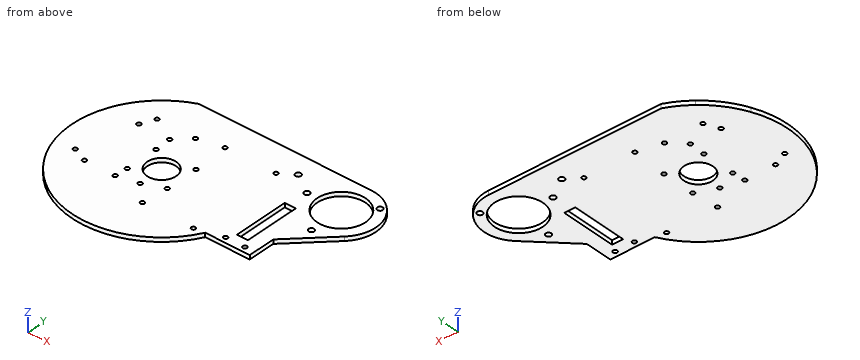
from build123d import *

# Parameters (mm, degrees)
SKETCH1_R           = 10.5
SKETCH1_R_2         = 1.5
SKETCH1_W           = 8
SKETCH1_H           = 40
SKETCH1_R_3         = 17.5
BOSS_EXTRUDE1_DEPTH = 3
CUT_EXTRUDE1_REACH  = 140.687
SKETCH2_R           = 2
CUT_EXTRUDE2_REACH  = 140.687
SKETCH3_R           = 2
BOSS_EXTRUDE2_START = -3
SKETCH4_R           = 65
SKETCH4_R_2         = 60
BOSS_EXTRUDE2_DEPTH = 3
CUT_EXTRUDE3_START  = -10
CUT_EXTRUDE3_DEPTH  = 10
CUT_EXTRUDE4_START  = -10
CUT_EXTRUDE4_DEPTH  = 10
CUT_EXTRUDE5_REACH  = 142.922
SKETCH7_R           = 1.5
CUT_EXTRUDE6_REACH  = 142.922
SKETCH8_R           = 1.5
CUT_EXTRUDE7_REACH  = 142.922
SKETCH9_R           = 1.5


with BuildPart() as part:
    # Sketch1 → Boss-Extrude1 (new body)
    # profile 1 of 2: a face of its own
    with BuildSketch(Plane.XY):
        with BuildLine():
            ThreePointArc((-60, 0), (-52.867640737, 28.372743309), (-33.166247904, 50))
            Line((-33.166247904, 50), (-60, 50))
            Line((-60, 50), (-60, 0))
        make_face()
    # profile 2 of 2: a face of its own
    with BuildSketch(Plane.XY):
        with BuildLine():
            ThreePointArc((0, 60), (-17.320508076, 57.445626465), (-33.166247904, 50))
            ThreePointArc((-33.166247904, 50), (-52.867640737, 28.372743309), (-60, 0))
            ThreePointArc((-60, 0), (-15.529142706, -57.955549577), (51.961524227, -30))
            Line((51.961524227, -30), (56.568542495, -30))
            Line((56.568542495, -30), (90, -30))
            Line((90, -30), (90, -10.355339059))
            Line((90, -10.355339059), (117.67766953, 17.32233047))
            ThreePointArc((117.67766953, 17.32233047), (123.096988313, 44.567085809), (100, 60))
            Line((100, 60), (0, 60))
        make_face()
        Circle(SKETCH1_R, mode=Mode.SUBTRACT)
        with Locations((69, -26)):
            Circle(SKETCH1_R_2, mode=Mode.SUBTRACT)
        with Locations((76, 0)):
            Rectangle(SKETCH1_W, SKETCH1_H, mode=Mode.SUBTRACT)
        with Locations((83, -26)):
            Circle(SKETCH1_R_2, mode=Mode.SUBTRACT)
        with Locations((100, 35)):
            Circle(SKETCH1_R_3, mode=Mode.SUBTRACT)
    extrude(amount=BOSS_EXTRUDE1_DEPTH)

    # Sketch2 → Cut-Extrude1 (cut, up to next)
    with BuildSketch(Plane.XY.offset(3), mode=Mode.PRIVATE) as cut_extrude1_sk1:
        with Locations((60, 45)):
            Circle(SKETCH2_R)
    cut_extrude1_tool1 = extrude(cut_extrude1_sk1.sketch, amount=-CUT_EXTRUDE1_REACH, mode=Mode.PRIVATE) & part.part
    add(cut_extrude1_tool1.solids().sort_by_distance((60, 45, 3))[0], mode=Mode.SUBTRACT)

    # Sketch3 → Cut-Extrude2 (cut, up to next)
    with BuildSketch(Plane.XY.offset(3), mode=Mode.PRIVATE) as cut_extrude2_sk1:
        with Locations((100, 10)):
            Circle(SKETCH3_R)
    cut_extrude2_tool1 = extrude(cut_extrude2_sk1.sketch, amount=-CUT_EXTRUDE2_REACH, mode=Mode.PRIVATE) & part.part
    # Sketch3 → Cut-Extrude2 (cut, up to next)
    with BuildSketch(Plane.XY.offset(3), mode=Mode.PRIVATE) as cut_extrude2_sk2:
        with Locations((75, 35)):
            Circle(SKETCH3_R)
    cut_extrude2_tool2 = extrude(cut_extrude2_sk2.sketch, amount=-CUT_EXTRUDE2_REACH, mode=Mode.PRIVATE) & part.part
    # Sketch3 → Cut-Extrude2 (cut, up to next)
    with BuildSketch(Plane.XY.offset(3), mode=Mode.PRIVATE) as cut_extrude2_sk3:
        with Locations((115.0260191, 50.0260191)):
            Circle(SKETCH3_R)
    cut_extrude2_tool3 = extrude(cut_extrude2_sk3.sketch, amount=-CUT_EXTRUDE2_REACH, mode=Mode.PRIVATE) & part.part
    add(cut_extrude2_tool1.solids().sort_by_distance((100, 10, 3))[0], mode=Mode.SUBTRACT)
    add(cut_extrude2_tool2.solids().sort_by_distance((75, 35, 3))[0], mode=Mode.SUBTRACT)
    add(cut_extrude2_tool3.solids().sort_by_distance((115.026019, 50.026019, 3))[0], mode=Mode.SUBTRACT)

    # Sketch4 → Boss-Extrude2 (add)
    with BuildSketch(Plane.XY.offset(3).offset(BOSS_EXTRUDE2_START)):
        Circle(SKETCH4_R)
        Circle(SKETCH4_R_2, mode=Mode.SUBTRACT)
    extrude(amount=BOSS_EXTRUDE2_DEPTH)

    # Sketch5 → Cut-Extrude3 (cut)
    with BuildSketch(Plane.XY.offset(3).offset(CUT_EXTRUDE3_START)):
        with BuildLine():
            Line((-60, 50), (-41.533119315, 50))
            ThreePointArc((-41.533119315, 50), (-52.282822987, 38.62002616), (-60, 25))
            Line((-60, 25), (-60, 50))
        make_face()
    extrude(amount=CUT_EXTRUDE3_DEPTH, mode=Mode.SUBTRACT)

    # Sketch6 → Cut-Extrude4 (cut)
    with BuildSketch(Plane.XY.offset(3).offset(CUT_EXTRUDE4_START)):
        with BuildLine():
            Line((25, 60), (-25, 60))
            ThreePointArc((-25, 60), (0, 65), (25, 60))
        make_face()
    extrude(amount=CUT_EXTRUDE4_DEPTH, mode=Mode.SUBTRACT)

    # Sketch7 → Cut-Extrude5 (cut, up to next)
    with BuildSketch(Plane.XY.offset(3), mode=Mode.PRIVATE) as cut_extrude5_sk1:
        with Locations((-14.5, 12)):
            Circle(SKETCH7_R)
    cut_extrude5_tool1 = extrude(cut_extrude5_sk1.sketch, amount=-CUT_EXTRUDE5_REACH, mode=Mode.PRIVATE) & part.part
    # Sketch7 → Cut-Extrude5 (cut, up to next)
    with BuildSketch(Plane.XY.offset(3), mode=Mode.PRIVATE) as cut_extrude5_sk2:
        with Locations((14.5, 12)):
            Circle(SKETCH7_R)
    cut_extrude5_tool2 = extrude(cut_extrude5_sk2.sketch, amount=-CUT_EXTRUDE5_REACH, mode=Mode.PRIVATE) & part.part
    # Sketch7 → Cut-Extrude5 (cut, up to next)
    with BuildSketch(Plane.XY.offset(3), mode=Mode.PRIVATE) as cut_extrude5_sk3:
        with Locations((-14.5, -12)):
            Circle(SKETCH7_R)
    cut_extrude5_tool3 = extrude(cut_extrude5_sk3.sketch, amount=-CUT_EXTRUDE5_REACH, mode=Mode.PRIVATE) & part.part
    # Sketch7 → Cut-Extrude5 (cut, up to next)
    with BuildSketch(Plane.XY.offset(3), mode=Mode.PRIVATE) as cut_extrude5_sk4:
        with Locations((14.5, -12)):
            Circle(SKETCH7_R)
    cut_extrude5_tool4 = extrude(cut_extrude5_sk4.sketch, amount=-CUT_EXTRUDE5_REACH, mode=Mode.PRIVATE) & part.part
    add(cut_extrude5_tool1.solids().sort_by_distance((-14.5, 12, 3))[0], mode=Mode.SUBTRACT)
    add(cut_extrude5_tool2.solids().sort_by_distance((14.5, 12, 3))[0], mode=Mode.SUBTRACT)
    add(cut_extrude5_tool3.solids().sort_by_distance((-14.5, -12, 3))[0], mode=Mode.SUBTRACT)
    add(cut_extrude5_tool4.solids().sort_by_distance((14.5, -12, 3))[0], mode=Mode.SUBTRACT)

    # Sketch8 → Cut-Extrude6 (cut, up to next)
    with BuildSketch(Plane.XY.offset(3), mode=Mode.PRIVATE) as cut_extrude6_sk1:
        with Locations((50, 38)):
            Circle(SKETCH8_R)
    cut_extrude6_tool1 = extrude(cut_extrude6_sk1.sketch, amount=-CUT_EXTRUDE6_REACH, mode=Mode.PRIVATE) & part.part
    # Sketch8 → Cut-Extrude6 (cut, up to next)
    with BuildSketch(Plane.XY.offset(3), mode=Mode.PRIVATE) as cut_extrude6_sk2:
        with Locations((13, 38)):
            Circle(SKETCH8_R)
    cut_extrude6_tool2 = extrude(cut_extrude6_sk2.sketch, amount=-CUT_EXTRUDE6_REACH, mode=Mode.PRIVATE) & part.part
    # Sketch8 → Cut-Extrude6 (cut, up to next)
    with BuildSketch(Plane.XY.offset(3), mode=Mode.PRIVATE) as cut_extrude6_sk3:
        with Locations((50, -31)):
            Circle(SKETCH8_R)
    cut_extrude6_tool3 = extrude(cut_extrude6_sk3.sketch, amount=-CUT_EXTRUDE6_REACH, mode=Mode.PRIVATE) & part.part
    # Sketch8 → Cut-Extrude6 (cut, up to next)
    with BuildSketch(Plane.XY.offset(3), mode=Mode.PRIVATE) as cut_extrude6_sk4:
        with Locations((13, -31)):
            Circle(SKETCH8_R)
    cut_extrude6_tool4 = extrude(cut_extrude6_sk4.sketch, amount=-CUT_EXTRUDE6_REACH, mode=Mode.PRIVATE) & part.part
    # Sketch8 → Cut-Extrude6 (cut, up to next)
    with BuildSketch(Plane.XY.offset(3), mode=Mode.PRIVATE) as cut_extrude6_sk5:
        with Locations((-5, 34)):
            Circle(SKETCH8_R)
    cut_extrude6_tool5 = extrude(cut_extrude6_sk5.sketch, amount=-CUT_EXTRUDE6_REACH, mode=Mode.PRIVATE) & part.part
    # Sketch8 → Cut-Extrude6 (cut, up to next)
    with BuildSketch(Plane.XY.offset(3), mode=Mode.PRIVATE) as cut_extrude6_sk6:
        with Locations((-32.9, 34)):
            Circle(SKETCH8_R)
    cut_extrude6_tool6 = extrude(cut_extrude6_sk6.sketch, amount=-CUT_EXTRUDE6_REACH, mode=Mode.PRIVATE) & part.part
    # Sketch8 → Cut-Extrude6 (cut, up to next)
    with BuildSketch(Plane.XY.offset(3), mode=Mode.PRIVATE) as cut_extrude6_sk7:
        with Locations((0.1, -18.1)):
            Circle(SKETCH8_R)
    cut_extrude6_tool7 = extrude(cut_extrude6_sk7.sketch, amount=-CUT_EXTRUDE6_REACH, mode=Mode.PRIVATE) & part.part
    # Sketch8 → Cut-Extrude6 (cut, up to next)
    with BuildSketch(Plane.XY.offset(3), mode=Mode.PRIVATE) as cut_extrude6_sk8:
        with Locations((-48.1, -16.8)):
            Circle(SKETCH8_R)
    cut_extrude6_tool8 = extrude(cut_extrude6_sk8.sketch, amount=-CUT_EXTRUDE6_REACH, mode=Mode.PRIVATE) & part.part
    add(cut_extrude6_tool1.solids().sort_by_distance((50, 38, 3))[0], mode=Mode.SUBTRACT)
    add(cut_extrude6_tool2.solids().sort_by_distance((13, 38, 3))[0], mode=Mode.SUBTRACT)
    add(cut_extrude6_tool3.solids().sort_by_distance((50, -31, 3))[0], mode=Mode.SUBTRACT)
    add(cut_extrude6_tool4.solids().sort_by_distance((13, -31, 3))[0], mode=Mode.SUBTRACT)
    add(cut_extrude6_tool5.solids().sort_by_distance((-5, 34, 3))[0], mode=Mode.SUBTRACT)
    add(cut_extrude6_tool6.solids().sort_by_distance((-32.9, 34, 3))[0], mode=Mode.SUBTRACT)
    add(cut_extrude6_tool7.solids().sort_by_distance((0.1, -18.1, 3))[0], mode=Mode.SUBTRACT)
    add(cut_extrude6_tool8.solids().sort_by_distance((-48.1, -16.8, 3))[0], mode=Mode.SUBTRACT)

    # Sketch9 → Cut-Extrude7 (cut, up to next)
    with BuildSketch(Plane.XY.offset(3), mode=Mode.PRIVATE) as cut_extrude7_sk1:
        with Locations((-15.055022894, 24)):
            Circle(SKETCH9_R)
    cut_extrude7_tool1 = extrude(cut_extrude7_sk1.sketch, amount=-CUT_EXTRUDE7_REACH, mode=Mode.PRIVATE) & part.part
    # Sketch9 → Cut-Extrude7 (cut, up to next)
    with BuildSketch(Plane.XY.offset(3), mode=Mode.PRIVATE) as cut_extrude7_sk2:
        with Locations((-15.055022894, -21.5)):
            Circle(SKETCH9_R)
    cut_extrude7_tool2 = extrude(cut_extrude7_sk2.sketch, amount=-CUT_EXTRUDE7_REACH, mode=Mode.PRIVATE) & part.part
    # Sketch9 → Cut-Extrude7 (cut, up to next)
    with BuildSketch(Plane.XY.offset(3), mode=Mode.PRIVATE) as cut_extrude7_sk3:
        with Locations((-37.355022894, 24)):
            Circle(SKETCH9_R)
    cut_extrude7_tool3 = extrude(cut_extrude7_sk3.sketch, amount=-CUT_EXTRUDE7_REACH, mode=Mode.PRIVATE) & part.part
    # Sketch9 → Cut-Extrude7 (cut, up to next)
    with BuildSketch(Plane.XY.offset(3), mode=Mode.PRIVATE) as cut_extrude7_sk4:
        with Locations((-37.355022894, -21.5)):
            Circle(SKETCH9_R)
    cut_extrude7_tool4 = extrude(cut_extrude7_sk4.sketch, amount=-CUT_EXTRUDE7_REACH, mode=Mode.PRIVATE) & part.part
    add(cut_extrude7_tool1.solids().sort_by_distance((-15.055023, 24, 3))[0], mode=Mode.SUBTRACT)
    add(cut_extrude7_tool2.solids().sort_by_distance((-15.055023, -21.5, 3))[0], mode=Mode.SUBTRACT)
    add(cut_extrude7_tool3.solids().sort_by_distance((-37.355023, 24, 3))[0], mode=Mode.SUBTRACT)
    add(cut_extrude7_tool4.solids().sort_by_distance((-37.355023, -21.5, 3))[0], mode=Mode.SUBTRACT)


solid = part.part
Could you check a few things on this model? Use its own coordinates, in mm. Coordinates: 2 decimals unless noted, no trailing zeros. Order: outer loops, then holes, each group sorted by start corner. A loop starts at its lowest first (then second) coordinate and runs counter-clockwise, first axis right, second up. Notation, with made-up numbers: (40.5, 73) -> (92.5, 73) arc R13 ccw to (92.5, 81) -> close; hole circle Ø8 at (41.5, 68.25). An arc over 180 degrees is marked (long way). One line per item, written item: value. Start each with the question number.
1) Imagine slicing it at C-C on z = 1.55. Count the separate pieces of the cut face and the enclosed holes in it, plus the area to 3 significant figures.
2) Imagine slicing it at D-D on x = -20. List the corners of the cut face in (y, z) for me, plus the area to 3 significant figures.
3) Imagine slicing it at B-B on y = 3.5. List the corners of the cut face in (x, z) for me.
4) If I drill on L1, parallel to Y at x = 0.1, z = 1.15; L2, parallel to Y at x = -6, z = 2.2; L3, parallel to X at y = 3, z = 2, over which ranges is the centre line in solid material (lowest first)? Write a range as [from, to].
5) Imagine slicing it at A-A on x = 60. List the corners of the cut face in (y, z) for me, plus the area to 3 significant figures.
6) I'm going to push flat-ended pins straight in: pin 1 (3.5 mm diameter, centred on x = -37.36, y = -21.5, fed in from -Z); pin 2 (1.5 mm diameter, centred on y = -21, z = 1, fed in from +X); pin 3 (1.5 mm diameter, centred on x = -18.5, z = 0.5, fed in from -Y); pin 4 (1 mm diameter, centred on x = 16, z = 2, fed in from -Y). Where does each tip first touch, or does it pass through?
Answer list:
1. separate pieces: 1
1. enclosed holes: 25
1. area: 16,000 mm2
2. outline: (-61.85, 0) -> (60, 0) -> (60, 3) -> (-61.85, 3) -> close
2. area: 366 mm2
3. outline: (-64.91, 0) -> (-9.9, 0) -> (-9.9, 3) -> (-64.91, 3) -> close; (9.9, 0) -> (72, 0) -> (72, 3) -> (9.9, 3) -> close; (80, 0) -> (103.86, 0) -> (103.86, 3) -> (80, 3) -> close
4. L1: y = [-65, -19.6], [-16.6, -10.5], [10.5, 60]
4. L2: y = [-64.72, -8.62], [8.62, 32.88], [35.12, 60]
4. L3: x = [-64.93, -10.06], [10.06, 72], [80, 103.36]
5. outline: (-30, 0) -> (43, 0) -> (43, 3) -> (-30, 3) -> close; (47, 0) -> (60, 0) -> (60, 3) -> (47, 3) -> close
5. area: 258 mm2
6. pin 1: stops at z = 0
6. pin 2: stops at x = 90
6. pin 3: stops at y = -62.53
6. pin 4: stops at y = -63.12
